Source: CAD feature listing. Evaluate the final solid. Frame: model axes, mm. Coordinates: 2 decimals unless noted, no trailing zeros. Order: outer loops, then holes, each group sorted by start corner. A loop starts at its lowest first (then second) coordinate and runs counter-clockwise, first axis right, second up. Notation, with made-up numbers: (34, -40) -> (74, -40) arc R14 ccw to (74, -20) -> close; hole circle Ø11 at (15.25, -12). An arc over 180 degrees is marked (long way). Put each result on its own line as item: value.
from build123d import *

# Parameters (mm, degrees)
SKETCH1_R           = 5
BOSS_EXTRUDE1_DEPTH = 10


with BuildPart() as part:
    # Sketch1 → Boss-Extrude1 (new body)
    with BuildSketch(Plane.XY):
        with BuildLine():
            ThreePointArc((-47.75, 14.83028995), (-65, 0), (-47.75, -14.83028995))
            ThreePointArc((-47.75, -14.83028995), (-43.301270189, -25), (-36.718407842, -33.937568056))
            ThreePointArc((-36.718407842, -33.937568056), (-32.5, -56.291651246), (-11.031592158, -48.767858006))
            ThreePointArc((-11.031592158, -48.767858006), (0, -50), (11.031592158, -48.767858006))
            ThreePointArc((11.031592158, -48.767858006), (32.5, -56.291651246), (36.718407842, -33.937568056))
            ThreePointArc((36.718407842, -33.937568056), (43.301270189, -25), (47.75, -14.83028995))
            ThreePointArc((47.75, -14.83028995), (65, 0), (47.75, 14.83028995))
            ThreePointArc((47.75, 14.83028995), (43.301270189, 25), (36.718407842, 33.937568056))
            ThreePointArc((36.718407842, 33.937568056), (32.5, 56.291651246), (11.031592158, 48.767858006))
            ThreePointArc((11.031592158, 48.767858006), (0, 50), (-11.031592158, 48.767858006))
            ThreePointArc((-11.031592158, 48.767858006), (-32.5, 56.291651246), (-36.718407842, 33.937568056))
            ThreePointArc((-36.718407842, 33.937568056), (-43.301270189, 25), (-47.75, 14.83028995))
        make_face()
        with Locations((-50, 0)):
            Circle(SKETCH1_R, mode=Mode.SUBTRACT)
        with Locations((-25, 43.301270189)):
            Circle(SKETCH1_R, mode=Mode.SUBTRACT)
        with Locations((25, 43.301270189)):
            Circle(SKETCH1_R, mode=Mode.SUBTRACT)
        with Locations((50, 0)):
            Circle(SKETCH1_R, mode=Mode.SUBTRACT)
        with Locations((25, -43.301270189)):
            Circle(SKETCH1_R, mode=Mode.SUBTRACT)
        with Locations((-25, -43.301270189)):
            Circle(SKETCH1_R, mode=Mode.SUBTRACT)
        with BuildLine():
            ThreePointArc((34.641016151, 20), (24.35045716, 31.734133612), (10.352761804, 38.637033052))
            ThreePointArc((10.352761804, 38.637033052), (4.229037447, 35.101499146), (7.764571353, 28.977774789))
            ThreePointArc((7.764571353, 28.977774789), (18.26284287, 23.800600209), (25.980762114, 15))
            ThreePointArc((25.980762114, 15), (32.810889132, 13.169872981), (34.641016151, 20))
        make_face(mode=Mode.SUBTRACT)
        with BuildLine():
            ThreePointArc((0, -40), (15.307337295, -36.9551813), (28.284271247, -28.284271247))
            ThreePointArc((28.284271247, -28.284271247), (28.284271247, -21.213203436), (21.213203436, -21.213203436))
            ThreePointArc((21.213203436, -21.213203436), (11.480502971, -27.716385975), (0, -30))
            ThreePointArc((0, -30), (-5, -35), (0, -40))
        make_face(mode=Mode.SUBTRACT)
        with BuildLine():
            ThreePointArc((-34.641016151, 20), (-39.657794455, 5.221047689), (-38.637033052, -10.352761804))
            ThreePointArc((-38.637033052, -10.352761804), (-32.513308695, -13.88829571), (-28.977774789, -7.764571353))
            ThreePointArc((-28.977774789, -7.764571353), (-29.743345841, 3.915785767), (-25.980762114, 15))
            ThreePointArc((-25.980762114, 15), (-27.810889132, 21.830127019), (-34.641016151, 20))
        make_face(mode=Mode.SUBTRACT)
    extrude(amount=BOSS_EXTRUDE1_DEPTH)


solid = part.part
1. Pull-direction query (X, two-part tool) for faces 1 (the cylindrical face through (11.633, -27.653, 4.93)), 2 (the cylindrical face through (24.525, 31.6, 4.93)); classes: pulls with the +X half, pulls with the -X half, needs draft (parallel to the pull), parting line crosses it, or undercut.
Numbers:
face 1: undercut
face 2: undercut
2. Cut plane D-D on x = 17.5. Output: boundary loops of the cut face in (y, z).
Numbers:
outline: (-56.29, 0) -> (-35.97, 0) -> (-35.97, 10) -> (-56.29, 10) -> close; (-24.37, 0) -> (24.37, 0) -> (24.37, 10) -> (-24.37, 10) -> close; (35.97, 0) -> (56.29, 0) -> (56.29, 10) -> (35.97, 10) -> close
3. Cut plane C-C on z = 4.25. Count the separate pieces of the cut face and the enclosed holes in it, plus the area to 3 significant figures.
Numbers:
separate pieces: 1
enclosed holes: 9
area: 8,580 mm2
4. First-contact query: pin 1 (1 mm diameter, centred on x = 12, z = 1, fed in from +Y); pin 2 (1.5 mm diameter, centred on x = -14.5, z = 5, fed in from +Y); pin 3 (9 mm diameter, centred on x = -25, y = -43.3, fed in from +Z); pin 4 (4 mm diameter, centred on x = 30, z = 5, fed in from -Y). Flat tips, straight axial feed; report the tip coordinate or a pass-through.
Numbers:
pin 1: stops at y = 51.59
pin 2: stops at y = 54.7
pin 3: passes through
pin 4: stops at y = -58
5. Ray query, line 1 along Y through (x, z) = (-25, 3); line 2 along Y through (x, z) = (-50, 6.25); line 3 along Y through (x, z) = (1, 5.75). Return the intervals inside material, ascending.
Numbers:
line 1: y = -58.3 to -48.3, -38.3 to 38.3, 48.3 to 58.3
line 2: y = -15 to -5, 5 to 15
line 3: y = -49.99 to -39.99, -29.98 to 49.99
6. Cut plane B-B on y = 18.5. Output: boundary loops of the cut face in (x, z).
Numbers:
outline: (-46.45, 0) -> (-35.46, 0) -> (-35.46, 10) -> (-46.45, 10) -> close; (-25.41, 0) -> (23.62, 0) -> (23.62, 10) -> (-25.41, 10) -> close; (35.21, 0) -> (46.45, 0) -> (46.45, 10) -> (35.21, 10) -> close
7. Cut plane A-A on x = -50. Output: boundary loops of the cut face in (y, z).
Numbers:
outline: (-15, 0) -> (-5, 0) -> (-5, 10) -> (-15, 10) -> close; (5, 0) -> (15, 0) -> (15, 10) -> (5, 10) -> close
